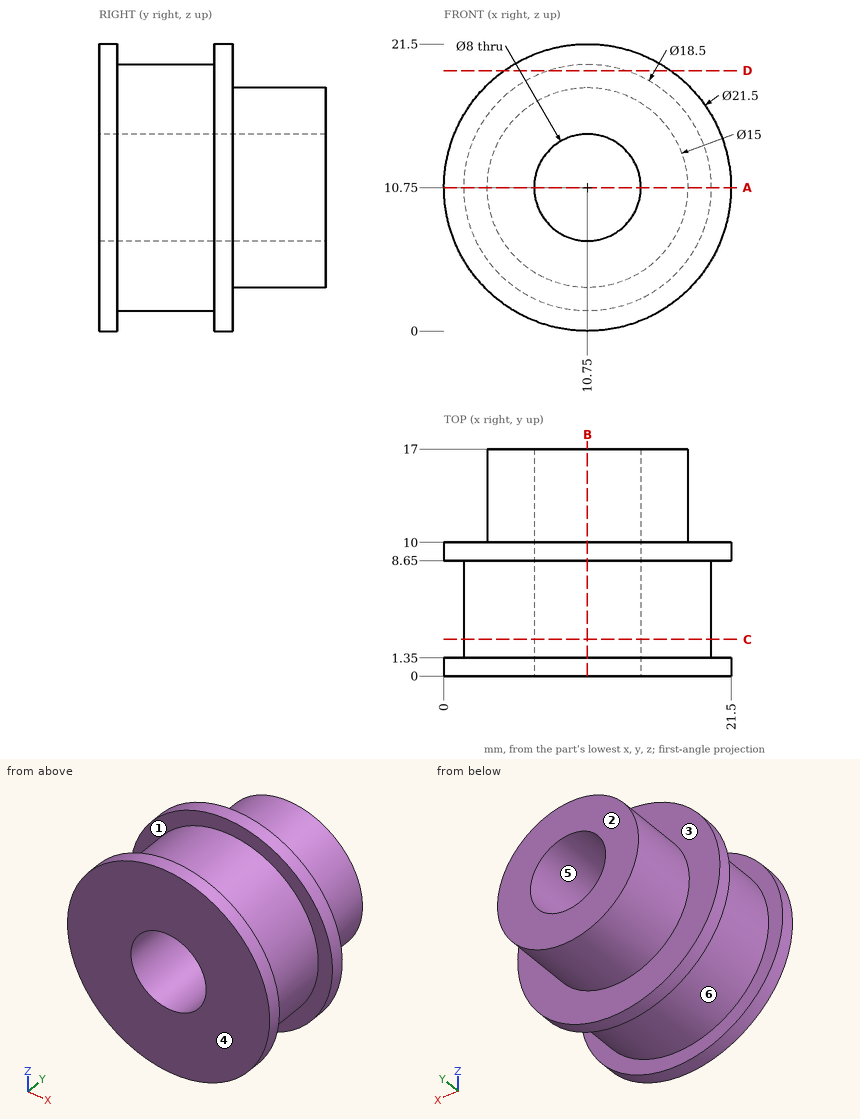
Print and shaded views of the part. All mm, measured from the part's lowest x, y and z. A direction names the side the tool comes from. Round coordinates to 2 decimals unless told otherwise and drop trailing zeros. Order: outer loops, then holes, each group sorted by start corner. A loop starts at its lowest first (then second) coordinate and runs counter-clockwise, first axis right, second up.
Q1. Slice it at B-B (x = 10.75). Write the cut outline in (y, z).
Q2. Slice it at C-C (y = 2.75). Write the cut outline in (x, z).
Q3. Slice it at A-A (z = 10.75). Write the cut outline in (x, y), and give its area (3 significant figures).
Q4. Two-plate mould, pull along Y, no slides. Class the marked faces 4, 5 and 6: pulls with the +Y half, pulls with the -Y half, needs draft (parallel to the pull), parting line crosses it, or undercut.
Q5. Slice it at D-D (z = 19.5). Write the cut outline in (x, y) (3 decimals), and give its area (3 significant figures).
Q6. Wall check: L1, parallel to X at y = 5.5, z = 10.75; L2, parallel to Y at x = 3.25, z = 4.75; L3, parallel to X at y = 16.25, z = 9.25. Give the ranges that are in metal, low to high.
Q7. Drop flat-ended pins along their axis: pin 1 (4 mm diameter, centred on x = 6.5, y = 5.5, fed in from -Z); pin 2 (2 mm diameter, centred on y = 14.5, z = 8, fed in from -X). Give the stop position or say it passes through.
Q8. Which spindle directions (+Z, -Z, +X, -X, +Y, -Y) get a long thin tool onto all of the face, cutting with end or side? Do the marked faces 1, 2 and 3. Say none if no direction does.
Results below:
1. outline: (0, 0) - (1.35, 0) - (1.35, 1.5) - (8.65, 1.5) - (8.65, 0) - (10, 0) - (10, 3.25) - (17, 3.25) - (17, 6.75) - (0, 6.75) - close; (0, 14.75) - (17, 14.75) - (17, 18.25) - (10, 18.25) - (10, 21.5) - (8.65, 21.5) - (8.65, 20) - (1.35, 20) - (1.35, 21.5) - (0, 21.5) - close
2. outline: circle Ø18.5 at (10.75, 10.75); hole circle Ø8 at (10.75, 10.75)
3. outline: (0, 0) - (6.75, 0) - (6.75, 17) - (3.25, 17) - (3.25, 10) - (0, 10) - (0, 8.65) - (1.5, 8.65) - (1.5, 1.35) - (0, 1.35) - close; (14.75, 0) - (21.5, 0) - (21.5, 1.35) - (20, 1.35) - (20, 8.65) - (21.5, 8.65) - (21.5, 10) - (18.25, 10) - (18.25, 17) - (14.75, 17) - close
3. area: 162 mm2
4. face 4: pulls with the -Y half
4. face 5: needs draft
4. face 6: undercut
5. outline: (4.505, 0) - (16.995, 0) - (16.995, 1.35) - (13.75, 1.35) - (13.75, 8.65) - (16.995, 8.65) - (16.995, 10) - (4.505, 10) - (4.505, 8.65) - (7.75, 8.65) - (7.75, 1.35) - (4.505, 1.35) - close
5. area: 77.5 mm2
6. L1: x = 1.5 to 6.75, 14.75 to 20
6. L2: y = 0 to 1.35, 8.65 to 10
6. L3: x = 3.4 to 7.04, 14.46 to 18.1
7. pin 1: stops at z = 1.78
7. pin 2: stops at x = 3.46
8. face 1: none
8. face 2: +Z, -Z, +X, -X, +Y
8. face 3: +Y
